Check sheet for the drawn part. Datum: minimum x, y, z corner. Units: mm. Give positions to 0.01 mm unless a question says otherwise; leave off trailing zeros. Loops run counter-clockwise (first coordinate to the right, second up) from the corner with the lowest first, then second, coordinate; pieces in that order, holes last.
1. Cross-section at D-D, the plane x = 56.5. Record the cut outline in (y, z).
2. Go/stop test with flat-tipped pins: pin 1 Ø4.5 at (x, z) = (12.09, 134.18) entering from +Y; pin 2 Ø1.5 at (x, y) = (181.5, 4.5) entering from -Z. Record where each tip stops, or that it passes through.
3. Release check for a two-part mould opening along Z. For the marked faces 1 and 2 record: +Z half, -Z half, draft (parallel to the pull), parting line (faces both ways), or undercut.
4. Cross-section at B-B, the plane z = 101.6. Record the cut outline in (x, y), plus the area to 3 significant figures.
5. Cross-section at A-A, the plane x = 101.6. Record the cut outline in (y, z).
6. Material ranges on L1, parallel to X at y = 2.75, z = 101.6; L2, parallel to Z at x = 183, y = 2.5 (1 decimal); L3, parallel to Z at x = 20.5, y = 0.5, recorded low to high.
7. Cross-section at C-C, the plane y = 1. State how many separate pieces and enclosed holes the cut face has, plus the area to 3 significant figures.
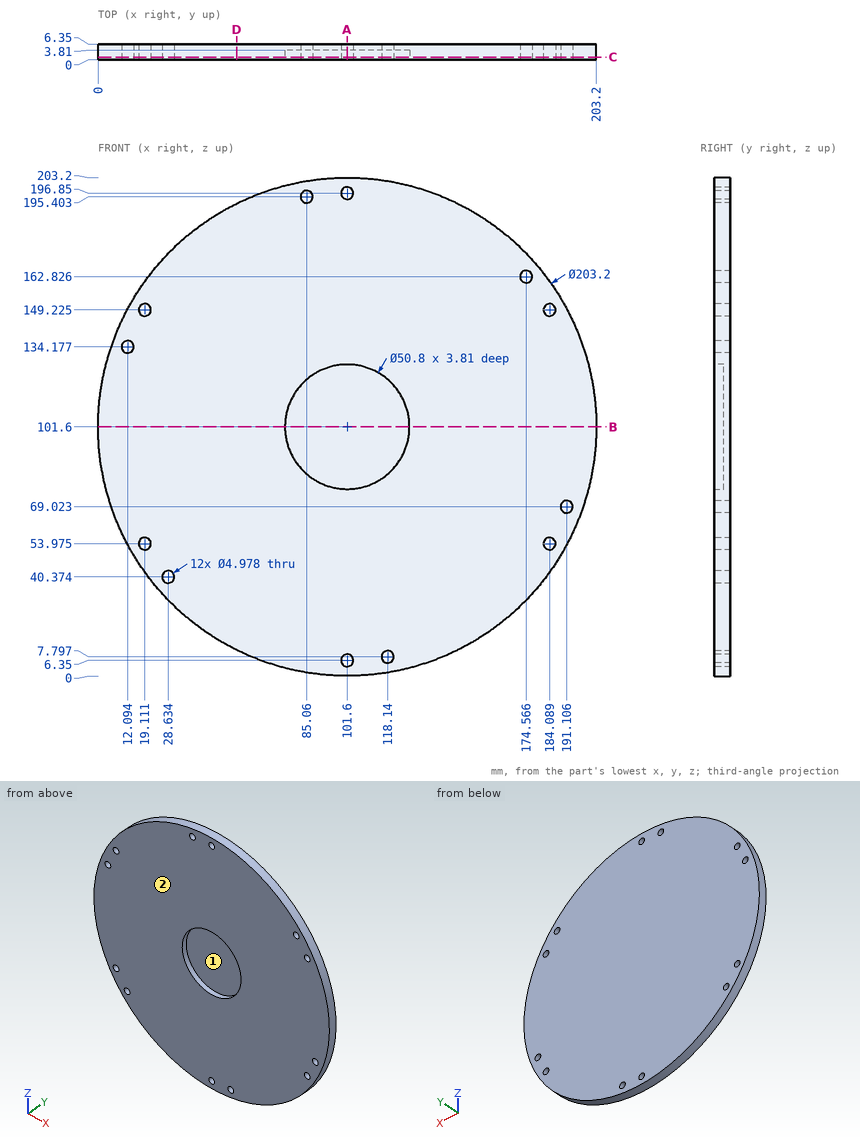
Result:
1. outline: (0, 10.56) - (6.35, 10.56) - (6.35, 192.64) - (0, 192.64) - close
2. pin 1: passes through
2. pin 2: stops at z = 37.9
3. face 1: undercut
3. face 2: draft
4. outline: (0, 0) - (76.2, 0) - (76.2, 3.81) - (127, 3.81) - (127, 0) - (203.2, 0) - (203.2, 6.35) - (0, 6.35) - close
4. area: 1,100 mm2
5. outline: (0, 0) - (6.35, 0) - (6.35, 3.86) - (0, 3.86) - close; (0, 8.84) - (6.35, 8.84) - (6.35, 194.36) - (0, 194.36) - (0, 127) - (3.81, 127) - (3.81, 76.2) - (0, 76.2) - close; (0, 199.34) - (6.35, 199.34) - (6.35, 203.2) - (0, 203.2) - close
6. L1: x = 0 to 76.2, 127 to 203.2
6. L2: z = 40.8 to 51.7, 56.2 to 147, 151.5 to 162.4
6. L3: z = 40.4 to 51.91, 56.04 to 147.16, 151.29 to 162.8
7. separate pieces: 1
7. enclosed holes: 13
7. area: 30,200 mm2
